Can you work these out from the model? Positions are in its coordinate system, mm. A direction names the side the tool comes from. Give positions to 0.01 mm unless a question says otherwise; leave off trailing zeros. Loops run counter-clockwise (first coordinate to the right, second up) from the corner with the lowest first, then second, coordinate; pieces in that order, holes last. Notation, with made-up numbers: (25.5, 81.25) - (52.5, 81.25) arc R10 ccw to (52.5, 86.25) - close; hole circle Ø1 at (-17.5, 51). An arc over 180 degrees is marked (long way). Answer in a Markdown table with one row per item.
from build123d import *

# Parameters (mm, degrees)
F1_DEPTH = 100
F2_R     = 5


with BuildPart() as f1:
    # F0 (on Front) → F1 (new body)
    with BuildSketch(Plane.XZ):
        Polygon((0, -200), (0, 0), (-100, 0), (-100, -300), (215, -300), (215, 700), (115, 700), (115, -200), align=None)
    extrude(amount=F1_DEPTH)

    # F2
    f2_edges = [f1.edges().sort_by_distance(p)[0] for p in [
        (-100, -100, -150),
        (115, -100, 250),
        (57.5, -100, -200),
        (0, -100, -100),
        (-50, -100, 0),
        (-100, -50, 0),
        (-100, 0, -150),
        (-100, -50, -300),
        (57.5, -100, -300),
        (57.5, 0, -300),
        (57.5, 0, -200),
        (0, 0, -100),
        (-50, 0, 0),
        (0, -50, 0),
        (115, 0, 250),
        (215, -50, -300),
        (215, -50, 700),
        (165, 0, 700),
        (165, -100, 700),
        (115, -50, 700),
        (215, 0, 200),
        (215, -100, 200),
    ]]
    fillet(f2_edges, radius=F2_R)


solid = f1.part
Q1. Imagine slicing it at B-B, the plane y = -74.5. Write out the boundary of the cut face in (x, z).
Checked values:
| item | result |
|---|---|
| outline | (-100, -295) arc R5 ccw to (-95, -300) - (210, -300) arc R5 ccw to (215, -295) - (215, 695) arc R5 ccw to (210, 700) - (120, 700) arc R5 ccw to (115, 695) - (115, -200) - (0, -200) - (0, -5) arc R5 ccw to (-5, 0) - (-95, 0) arc R5 ccw to (-100, -5) - close |
Q2. If we mould it in two halves opening along X, with no side actions, what happens to faces 4 (the face through (55, -49, -300)), 5 (the face through (215, -49, 193)), 6 (the face through (0, -49, -104))? For each: released by +X, released by -X, zero draft, split by the parting line, or undercut.
Checked values:
| item | result |
|---|---|
| face 4 | zero draft |
| face 5 | released by +X |
| face 6 | undercut |
Q3. On a 3-axis mill with a long thin cutter (end or side, diameter ignored), from which of +Z, -Z, +X, -X, +Y, -Y can I reach the whole of each face in a straight line? I mean faces 1 (the face through (58, -49, -200)), 2 (the face through (-49, -49, 0)), 3 (the face through (-100, -49, -148)). Say none if no direction works.
Checked values:
| item | result |
|---|---|
| face 1 | +Z, +Y, -Y |
| face 2 | +Z, -X, +Y, -Y |
| face 3 | +Z, -Z, -X, +Y, -Y |
Q4. If I drill on line 1 (X direction, y = -8.5, z = -61.5); line 2 (X direction, y = -75, z = 129.5); line 3 (Z direction, x = -47, y = -68), over which ranges is the centre line in solid material (lowest first)? Write a range as [from, to].
Checked values:
| item | result |
|---|---|
| line 1 | x = [-100, 0], [115, 215] |
| line 2 | x = [115, 215] |
| line 3 | z = [-300, 0] |
Q5. Imagine slicing it at C-C, the plane z = 593.5. Write out the boundary of the cut face in (x, y), and give its area (3 significant figures).
Checked values:
| item | result |
|---|---|
| outline | (115, -95) arc R5 ccw to (120, -100) - (210, -100) arc R5 ccw to (215, -95) - (215, -5) arc R5 ccw to (210, 0) - (120, 0) arc R5 ccw to (115, -5) - close |
| area | 9,980 mm² |
Q6. Imagine slicing it at A-A, the plane x = 74.5. Write out the boundary of the cut face in (y, z).
Checked values:
| item | result |
|---|---|
| outline | (-100, -295) arc R5 ccw to (-95, -300) - (-5, -300) arc R5 ccw to (0, -295) - (0, -205) arc R5 ccw to (-5, -200) - (-95, -200) arc R5 ccw to (-100, -205) - close |
Q7. For pin 1 (12 mm diameter, centred on x = 76, y = -40, fed in from +Z); pin 2 (5 mm diameter, centred on y = -40, z = 494.5, fed in from -X), each with a flat end and sliding along its axis, tell me the tip position at first contact or that it passes through.
Checked values:
| item | result |
|---|---|
| pin 1 | stops at z = -200 |
| pin 2 | stops at x = 115 |
